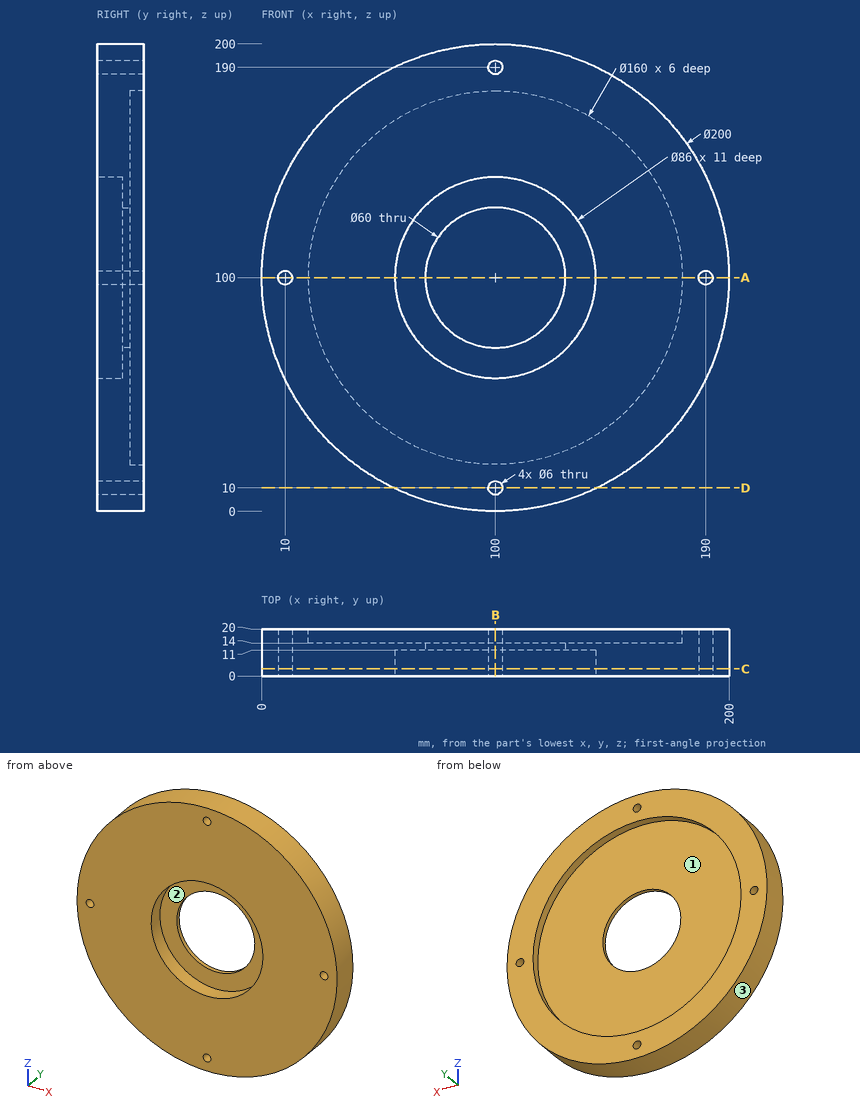
For this review, use the dimensioned drawing (mm, ordinates from the lowest corner) and the shaded views. Give positions to 0.01 mm unless a question says otherwise; leave off trailing zeros. Write each loop counter-clockwise with the first axis right and the second up, starting at its lowest first coordinate (ties: lowest second). Pieces come first, ordered by that corner, then holes. Notation, with made-up numbers: M 33,23.25 L 47,23.25 A15 ccw 47,47.25 Z; hole C 32.25,-32.75 d5. An arc over 180 degrees is marked long. Answer as a JSON object with one key per item and string values. Group by question number.
1) Clearance check with flat-ended pins moving along their axes: pin 1 Ø5 at (x, z) = (10, 100) entering from -Y; pin 2 Ø9.5 at (x, z) = (100, 10) entering from -Y; pin 3 Ø6 at (y, z) = (17, 136) entering from +X; pin 4 Ø10 at (x, z) = (137.5, 76.5) entering from +Y. State where each tip first meets the part, or that it passes through.
2) We need section D-D (z = 10). Give the boundary of the cut face in (x, y), and give its area (3 significant figures).
3) For line 1 along X through (y, z) = (12.25, 100); line 2 along X through (y, z) = (6.75, 100); line 3 along Y through (x, z) = (43, 111), list the stretches that pass through material, from the lowest coordinate up.
4) We need section B-B (x = 100). Give the boundary of the cut face in (y, z).
5) We need section A-A (z = 100). Give the boundary of the cut face in (x, y), and give its area (3 significant figures).
6) Mouldability with a two-part tool opening along Y and no side actions: class the marked faces 1, 2 and 3 as released by +Y, released by -Y, zero draft, split by the parting line, or undercut.
7) We need section C-C (y = 3). Give the boundary of the cut face in (x, z), and give its area (3 significant figures).
Answer key:
{
 "1": {"pin 1": "passes through", "pin 2": "stops at y = 0", "pin 3": "stops at x = 194.4", "pin 4": "stops at y = 14"},
 "2": {"outline": "M 56.41,0 L 97,0 L 97,20 L 56.41,20 Z; M 103,0 L 143.59,0 L 143.59,20 L 103,20 Z", "area": "1,620 mm²"},
 "3": {"line 1": "x = 0 to 7, 13 to 70, 130 to 187, 193 to 200", "line 2": "x = 0 to 7, 13 to 57, 143 to 187, 193 to 200", "line 3": "y = 0 to 14"},
 "4": {"outline": "M 0,0 L 20,0 L 20,7 L 0,7 Z; M 0,13 L 20,13 L 20,20 L 14,20 L 14,70 L 11,70 L 11,57 L 0,57 Z; M 0,143 L 11,143 L 11,130 L 14,130 L 14,180 L 20,180 L 20,187 L 0,187 Z; M 0,193 L 20,193 L 20,200 L 0,200 Z"},
 "5": {"outline": "M 0,0 L 7,0 L 7,20 L 0,20 Z; M 13,0 L 57,0 L 57,11 L 70,11 L 70,14 L 20,14 L 20,20 L 13,20 Z; M 130,11 L 143,11 L 143,0 L 187,0 L 187,20 L 180,20 L 180,14 L 130,14 Z; M 193,0 L 200,0 L 200,20 L 193,20 Z", "area": "1,670 mm²"},
 "6": {"face 1": "released by +Y", "face 2": "released by -Y", "face 3": "zero draft"},
 "7": {"outline": "C 100,100 d200; hole C 10,100 d6; hole C 100,100 d86; hole C 100,10 d6; hole C 100,190 d6; hole C 190,100 d6", "area": "25,500 mm²"}
}
